from build123d import *

# Parameters (mm, degrees)
SM_BASE_FLANGE_1_DEPTH             = 1
SM_EDGE_FLANGE_1_STRIP_W           = 6
SM_EDGE_FLANGE_1_STRIP_H           = 1
SM_EDGE_FLANGE_1_STRIP_CUT_DEPTH   = 160
SM_EDGE_FLANGE_1_DEPTH             = 160
SM_EDGE_FLANGE_2_STRIP_W           = 6
SM_EDGE_FLANGE_2_STRIP_H           = 1
SM_EDGE_FLANGE_2_STRIP_CUT_DEPTH   = 66.5
SM_EDGE_FLANGE_2_STRIP_2_W         = 6
SM_EDGE_FLANGE_2_STRIP_2_H         = 1
SM_EDGE_FLANGE_2_STRIP_CUT_2_DEPTH = 66.5
SM_EDGE_FLANGE_2_DEPTH             = 66.5
SM_EDGE_FLANGE_2_BEND_DEPTH        = 66.5
SKETCH_15_R                        = 1.75
CUT_EXTRUDE_1_DEPTH                = 10
FILLET_1_R                         = 4
SKETCH_16_R                        = 2.1
CUT_EXTRUDE_2_DEPTH                = 213.438814721


# Sheet-metal steps are written as plain solids
with BuildPart() as part:
    # Sketch 1 → Базовая кромка1 (new body)
    with BuildSketch(Plane(origin=(0, 0, 0), x_dir=(1, 0, 0), z_dir=(0, 1, 0))):
        Polygon((0, 0), (66.5, 0), (66.5, -14), (94.5, -14), (94.5, -174), (66.5, -174), (66.5, -188), (0, -188), align=None)
    extrude(amount=-SM_BASE_FLANGE_1_DEPTH)

    # Ребро-кромка1 strip (across the edge) → Ребро-кромка1 strip cut (cut)
    with BuildSketch(Plane(origin=(94.5, -1, 14), x_dir=(-1, 0, 0), z_dir=(0, 0, 1))):
        with Locations((-1, -0.5)):
            Rectangle(SM_EDGE_FLANGE_1_STRIP_W, SM_EDGE_FLANGE_1_STRIP_H)
    extrude(amount=SM_EDGE_FLANGE_1_STRIP_CUT_DEPTH, mode=Mode.SUBTRACT)

    # Ребро-кромка1 section (across the edge) → Ребро-кромка1 (add)
    with BuildSketch(Plane(origin=(94.5, -1, 14), x_dir=(-1, 0, 0), z_dir=(0, 0, 1))):
        with BuildLine():
            Line((0, 1), (0, 9))
            Line((0, 9), (1, 9))
            Line((1, 9), (1, 1))
            ThreePointArc((1, 1), (1.292893219, 0.292893219), (2, 0))
            Line((2, 0), (2, -1))
            ThreePointArc((2, -1), (0.585786438, -0.414213562), (0, 1))
        make_face()
    extrude(amount=SM_EDGE_FLANGE_1_DEPTH)

    # Ребро-кромка2 strip (across the edge) → Ребро-кромка2 strip cut (cut)
    with BuildSketch(Plane(origin=(66.5, -1, 188), x_dir=(0, 0, -1), z_dir=(-1, 0, 0))):
        with Locations((-2, -0.5)):
            Rectangle(SM_EDGE_FLANGE_2_STRIP_W, SM_EDGE_FLANGE_2_STRIP_H)
    extrude(amount=SM_EDGE_FLANGE_2_STRIP_CUT_DEPTH, mode=Mode.SUBTRACT)

    # Ребро-кромка2 strip 2 (across the edge) → Ребро-кромка2 strip cut 2 (cut)
    with BuildSketch(Plane(origin=(0, -1, 0), x_dir=(0, 0, 1), z_dir=(1, 0, 0))):
        with Locations((-2, -0.5)):
            Rectangle(SM_EDGE_FLANGE_2_STRIP_2_W, SM_EDGE_FLANGE_2_STRIP_2_H)
    extrude(amount=SM_EDGE_FLANGE_2_STRIP_CUT_2_DEPTH, mode=Mode.SUBTRACT)

    # Ребро-кромка2 section (across the edge) → Ребро-кромка2 (add)
    with BuildSketch(Plane(origin=(66.5, -1, 188), x_dir=(0, 0, -1), z_dir=(-1, 0, 0))):
        with BuildLine():
            Line((-1, 1), (-1, 9))
            Line((-1, 9), (0, 9))
            Line((0, 9), (0, 1))
            ThreePointArc((0, 1), (0.292893219, 0.292893219), (1, 0))
            Line((1, 0), (1, -1))
            ThreePointArc((1, -1), (-0.414213562, -0.414213562), (-1, 1))
        make_face()
    extrude(amount=SM_EDGE_FLANGE_2_DEPTH)

    # Ребро-кромка2 section 2 (across the edge) → Ребро-кромка2 bend (add)
    with BuildSketch(Plane(origin=(0, -1, 0), x_dir=(0, 0, 1), z_dir=(1, 0, 0))):
        with BuildLine():
            Line((-1, 1), (-1, 9))
            Line((-1, 9), (0, 9))
            Line((0, 9), (0, 1))
            ThreePointArc((0, 1), (0.292893219, 0.292893219), (1, 0))
            Line((1, 0), (1, -1))
            ThreePointArc((1, -1), (-0.414213562, -0.414213562), (-1, 1))
        make_face()
    extrude(amount=SM_EDGE_FLANGE_2_BEND_DEPTH)

    # Эскиз15 → Вырез-Вытянуть1 (cut)
    with BuildSketch(Plane(origin=(94.5, 0, 0), x_dir=(0, 0, -1), z_dir=(1, 0, 0))):
        with Locations(Location((-168, -6, 0), (0, 0, 90))):
            Circle(SKETCH_15_R)
        with Locations(Location((-20, -6, 0), (0, 0, 90))):
            Circle(SKETCH_15_R)
    extrude(amount=-CUT_EXTRUDE_1_DEPTH, mode=Mode.SUBTRACT)

    # Скругление1
    fillet_1_edges = [part.edges().sort_by_distance(p)[0] for p in [
        (0, -10, -0.5),
        (66.5, -10, -0.5),
        (66.5, -0.5, 14),
        (66.5, -0.5, 174),
        (94, -10, 14),
        (94, -10, 174),
        (66.5, -10, 188.5),
        (0, -10, 188.5),
    ]]
    fillet(fillet_1_edges, radius=FILLET_1_R)

    # Эскиз16 → Вырез-Вытянуть2 (cut, through all)
    with BuildSketch(Plane.XY.offset(189)):
        with Locations((5, -7)):
            Circle(SKETCH_16_R)
        with Locations((60, -7)):
            Circle(SKETCH_16_R)
    extrude(amount=-CUT_EXTRUDE_2_DEPTH, mode=Mode.SUBTRACT)


solid = part.part
Geometry check sheet. Reference: the model listing, model coordinates, mm. A direction names the side the tool comes from. Give positions to 0.01 mm unless a question says otherwise; leave off trailing zeros. Write each loop counter-clockwise with the first axis right and the second up, starting at its lowest first coordinate (ties: lowest second). Pieces come first, ordered by that corner, then holes. Notation, with made-up numbers: (34, 76.25) - (63, 76.25) arc R16 ccw to (63, 93.25) - close; hole circle Ø3 at (18, -11.75). An arc over 180 degrees is marked (long way). Put each result on its own line as item: value.
1. Set-up check for faces 5 (the cylindrical face through (65.297, -8.859, -0.493)), 6 (the flat face through (47, -1, 93)), 7 (the flat face through (33, -6, 0)), 8 (the flat face through (66.5, -0.8, 184.7)), 9 (the flat face through (93.5, -6, 93)): record each of +Z, -Z, +X, -X, +Y, -Y from which the full face is reachable in a straight line by a thin tool's end or side.
Ans:
face 5: +Z, -Z, +X, -Y
face 6: -X, -Y
face 7: +X, -X, -Y
face 8: +Z, +X, +Y, -Y
face 9: +Z, -Z, -X, -Y
2. Sectioned sample at C-C, the plane z = 153. Enter the section's corners in (x, y), plus the area to 3 significant figures.
Ans:
outline: (0, -1) - (92.5, -1) arc R1 cw to (93.5, -2) - (93.5, -10) - (94.5, -10) - (94.5, -2) arc R2 ccw to (92.5, 0) - (0, 0) - close
area: 103 mm²
3. Sectioned sample at A-A, the plane z = 20. Enter the section's corners in (x, y).
Ans:
outline: (0, -1) - (92.5, -1) arc R1 cw to (93.5, -2) - (93.5, -4.25) - (94.5, -4.25) - (94.5, -2) arc R2 ccw to (92.5, 0) - (0, 0) - close; (93.5, -10) - (94.5, -10) - (94.5, -7.75) - (93.5, -7.75) - close
4. Sectioned sample at B-B, the plane x = 60. Enter the section's corners in (y, z), plus the area to 3 significant figures.
Ans:
outline: (-10, -1) - (-9.1, -1) - (-9.1, 0) - (-10, 0) - close; (-10, 188) - (-9.1, 188) - (-9.1, 189) - (-10, 189) - close; (-4.9, -1) - (-2, -1) arc R2 ccw to (0, 1) - (0, 187) arc R2 ccw to (-2, 189) - (-4.9, 189) - (-4.9, 188) - (-2, 188) arc R1 cw to (-1, 187) - (-1, 1) arc R1 cw to (-2, 0) - (-4.9, 0) - close
area: 198 mm²
5. Go/stop test with flat-tipped pins: pin 1 (8 mm diameter, centred on x = 57.5, z = 34.5, fed in from +Y); pin 2 (3 mm diameter, centred on x = 84.5, y = -1.5, fed in from +Z); pin 3 (6 mm diameter, centred on x = 39.5, z = 98, fed in from -Y); pin 4 (2 mm diameter, centred on y = -3.5, z = 44.5, fed in from -X). Record where each tip stops, or that it passes through.
Ans:
pin 1: stops at y = 0
pin 2: stops at z = 174
pin 3: stops at y = -1
pin 4: stops at x = 93.5
6. Draft check along Z on faces 1 (the flat face through (84.2, -0.8, 174)), 2 (the flat face through (33, -6, -1)), 3 (the flat face through (34, -6, 188)), 4 (the cylindrical face through (4.727, -4.918, 188.507)). Enter one of: +Z half, -Z half, draft (parallel to the pull), parting line (faces both ways), or undercut.
Ans:
face 1: +Z half
face 2: -Z half
face 3: undercut
face 4: draft
7. Thickness scan on line 1 (Z direction, x = 94.2, y = -6); line 2 (Z direction, x = 47, y = -9.25); line 3 (Y direction, x = 78, z = 120). Record the ranges inside material, lowest first.
Ans:
line 1: z = 14 to 18.25, 21.75 to 166.25, 169.75 to 174
line 2: z = -1 to 0, 188 to 189
line 3: y = -1 to 0
8. Sectioned sample at D-D, the plane x = 86. Enter the section's corners in (y, z).
Ans:
outline: (-1, 14) - (0, 14) - (0, 174) - (-1, 174) - close
